Work out the finished part from the listing and answer in its coordinate system (mm). Coordinates: 2 decimals unless noted, no trailing zeros. Order: outer loops, then holes, each group sorted by start corner. A loop starts at its lowest first (then second) coordinate and runs counter-clockwise, first axis right, second up. Notation, with made-up numbers: (3.25, -8.75) - (16.25, -8.75) arc R18 ccw to (16.25, -0.75) - close; hole circle Ø6 at (81, 36). An arc over 180 degrees is marked (long way). Answer as a JSON object with one key per item and string values. Group by question number.
1) Section B-B (x = -0.6) is taken. Give the vertices of the cut face in (y, z), plus the area to 3 significant figures.
2) Section C-C (y = -74) is taken. Give the vertices of the cut face in (x, z), plus the area to 3 significant figures.
3) Section D-D (z = 204) is taken. Give the vertices of the cut face in (x, y), plus the area to 3 significant figures.
4) Section A-A (z = 110.5) is taken. Give the vertices of the cut face in (x, y), plus the area to 3 significant figures.
5) Find the intervals of material crossed by line 1 along Y through (x, z) = (-0.9, 93); line 2 along Y through (x, z) = (0.85, 76.5); line 3 along Z through (x, y) = (-0.1, -110), in increasing order.
6) Each of these flat-tipped pins is pushed along its axis until it touches: P1, Ø1, axis at x = -1, z = 128, coming from the +Y side; P2, Ø0.9, axis at x = -0.5, z = 112, coming from the +Y side (3 decimals). Where does it stop, or does it pass through?
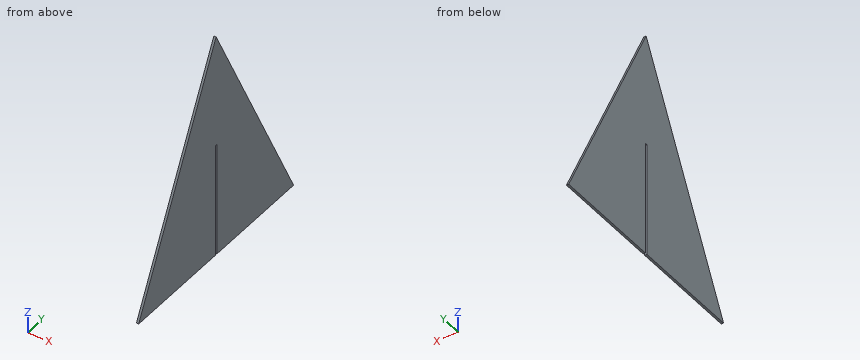
Autodesk Inventor part; units mm, degrees
ref_plane "YZ Plane" through (0, 0, 0) normal (1, 0, 0) x (0, 1, 0)
ref_plane "XZ Plane" through (0, 0, 0) normal (0, 1, 0) x (-1, 0, 0)
ref_plane "XY Plane" through (0, 0, 0) normal (0, 0, 1) x (1, 0, 0)
sketch "Sketch1" plane through (0, 0, 0) normal (1, 0, 0) x (0, 1, 0)
  line L0 (150, 0) -> (-150, 0)
  line L1 (0, 0) -> (0, 300)
  line L2 (0, 300) -> (150, 0)
  line L3 (0, 300) -> (-150, 0)
  dimension "d0" = 300
  dimension "d1" = 300
extrude "Plate1" add sketch "Sketch1" along normal mid plane 3
sketch "Sketch3" plane through (1.5, 0, 0) normal (1, 0, 0) x (0, 0, -1)
  line L0 (0, -1.6) -> (-151, -1.6)
  line L1 (-151, -1.6) -> (-151, 1.6)
  line L2 (-151, 1.6) -> (0, 1.6)
  line L3 (0, 1.6) -> (0, -1.6)
  line L4 (0, 150) -> (0, -150)
  point P0 (0, 0)
  point P1 (0, 0)
  dimension "d7" = 3.2
  dimension "d8" = 151
extrude "Extrusion2" cut sketch "Sketch3" against normal through all
equation "\"d2\" = Thickness"
equation "\"BendReliefWidth\" = Thickness"
equation "\"BendReliefDepth\" = 0.5 * Thickness"
equation "\"CornerReliefSize\" = 4 * Thickness"
equation "\"MinimumRemnant\" = 2 * Thickness"
equation "\"TransitionRadius\" = BendRadius"
equation "\"JacobiRadiusSize\" = BendRadius"
equation "\"GapSize\" = Thickness"
properties part number "MSC 207 CONE BLADE" material "Stainless Steel"
Report:
{
 "1": {"outline": "(-150, 0) - (-1.6, 0) - (-1.6, 151) - (1.6, 151) - (1.6, 0) - (150, 0) - (0, 300) - close", "area": "44,500 mm²"},
 "2": {"outline": "(-1.5, 0) - (1.5, 0) - (1.5, 152) - (-1.5, 152) - close", "area": "456 mm²"},
 "3": {"outline": "(-1.5, -48) - (1.5, -48) - (1.5, 48) - (-1.5, 48) - close", "area": "288 mm²"},
 "4": {"outline": "(-1.5, -94.75) - (1.5, -94.75) - (1.5, -1.6) - (-1.5, -1.6) - close; (-1.5, 1.6) - (1.5, 1.6) - (1.5, 94.75) - (-1.5, 94.75) - close", "area": "559 mm²"},
 "5": {"line 1": "y = -103.5 to -1.6, 1.6 to 103.5", "line 2": "y = -111.75 to -1.6, 1.6 to 111.75", "line 3": "z = 0 to 80"},
 "6": {"P1": "stops at y = 86.25", "P2": "stops at y = 94.225"}
}
